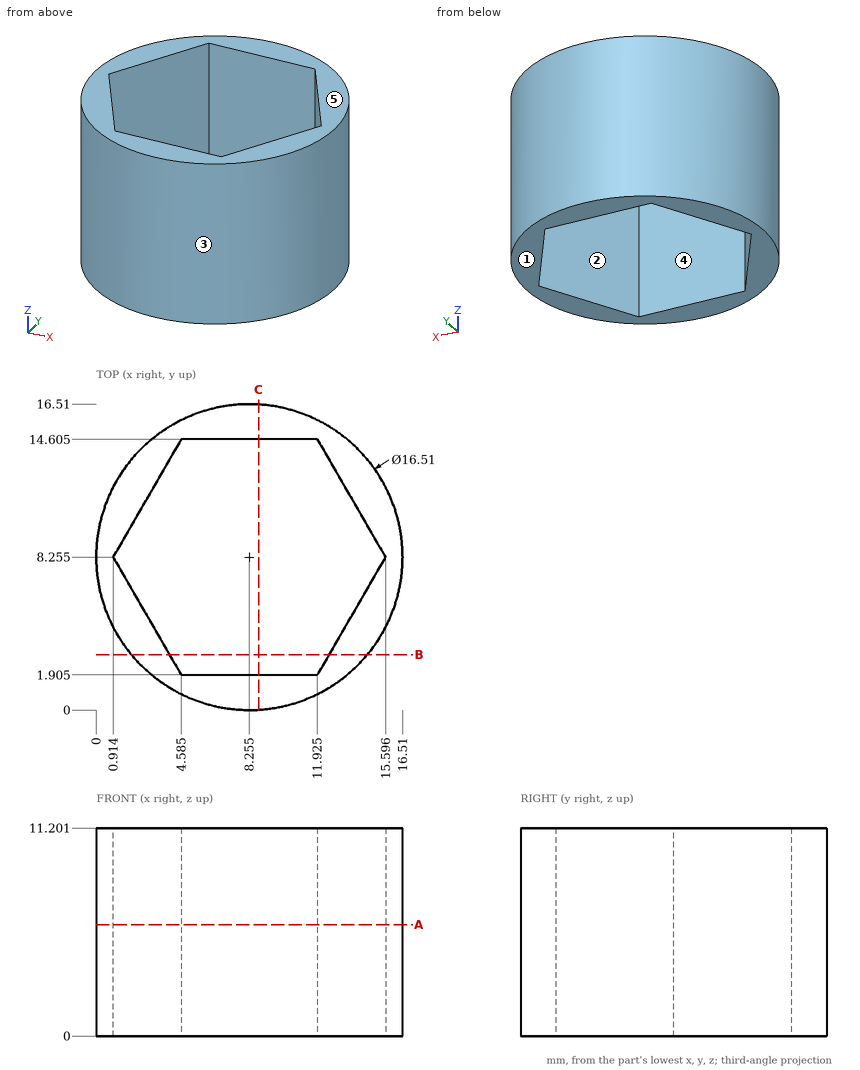
Design review of the part shown in the three views and the two pictorial views. Dimensions are in mm from the part's minimum x, y and z. A direction names the side the tool comes from. Give positions to 0.01 mm unless a question says otherwise; leave off trailing zeros. Loops run counter-clockwise (first coordinate to the right, second up) from the corner with the lowest first, then second, coordinate; pieces in that order, holes last. Notation, with made-up numbers: (-23.5, 36) - (18.5, 36) arc R23 cw to (18.5, 75) - close; hole circle Ø7 at (-35, 74.5). An arc over 180 degrees is marked (long way). Write item = value, one per line.
1) To check wall thickness, follow line 1 (X direction, y = 6.75, z = 9.5) (1 decimal); line 2 (X direction, y = 3.75, z = 8.5); line 3 (Y direction, x = 3.25, z = 10.75) (1 decimal). State the ranges of each line that lie inside material, in increasing order.
Result sheet:
line_1 = 0.1 to 1.8, 14.7 to 16.4
line_2 = 1.34 to 3.52, 12.99 to 15.17
line_3 = 1.7 to 4.2, 12.3 to 14.8
2) Clearance check with flat-ended pins moving along their axes: pin 1 Ø1 at (x, z) = (10, 8) entering from +Y (1 decimal); pin 2 Ø4 at (x, z) = (13.5, 1.5) entering from +Y (1 decimal); pin 3 Ø1.5 at (y, z) = (10.5, 6) entering from +X. State where each tip first meets the part, or that it passes through.
Result sheet:
pin_1 = 16.4
pin_2 = 15.8
pin_3 = 16.37
3) Take a section at A-A on z = 6. State the section outline as (x, y) points (1 decimal).
Result sheet:
outline = circle Ø16.5 at (8.3, 8.3); hole (0.9, 8.3) - (4.6, 1.9) - (11.9, 1.9) - (15.6, 8.3) - (11.9, 14.6) - (4.6, 14.6) - close
4) Draft analysis for pull direction Y (two halves, no side actions). For the marked faces 1, 2 and 3, state which applies: +Y half, -Y half, draft (parallel to the pull), parting line (faces both ways), or undercut.
Result sheet:
face_1 = draft
face_2 = undercut
face_3 = parting line
5) Take a section at C-C on x = 8.75. State the section outline as (y, z) points (1 decimal).
Result sheet:
outline = (0, 0) - (1.9, 0) - (1.9, 11.2) - (0, 11.2) - close; (14.6, 0) - (16.5, 0) - (16.5, 11.2) - (14.6, 11.2) - close
6) Tool access review of the marked faces 4 and 5: name each direction out of +Z, -Z, +X, -X, +Y, -Y from which nothing blocks a thin tool from reaching the whole face with its end or side.
Result sheet:
face_4 = +Z, -Z
face_5 = +Z, +X, -X, +Y, -Y
7) Take a section at B-B on y = 3. State the section outline as (x, z) points.
Result sheet:
outline = (1.89, 0) - (3.95, 0) - (3.95, 11.2) - (1.89, 11.2) - close; (12.56, 0) - (14.62, 0) - (14.62, 11.2) - (12.56, 11.2) - close
